Autodesk Inventor part; units mm, degrees
ref_plane "YZ Plane" through (0, 0, 0) normal (1, 0, 0) x (0, 1, 0)
ref_plane "XZ Plane" through (0, 0, 0) normal (0, 1, 0) x (-1, 0, 0)
ref_plane "XY Plane" through (0, 0, 0) normal (0, 0, 1) x (1, 0, 0)
sketch "Sketch1" plane through (0, 0, 0) normal (1, 0, 0) x (0, 1, 0)
  line L0 (0, 0) -> (800, 0)
  line L1 (800, 0) -> (800, -750)
  line L2 (800, -750) -> (0, -750)
  line L3 (0, -750) -> (0, 0)
  dimension "d0" = 800
  dimension "d1" = 750
extrude "Extrusion1" add sketch "Sketch1" along normal blind 18
sketch "Sketch2" plane through (18, 0, 0) normal (1, 0, 0) x (0, 0, -1)
  line L0 (0, 800) -> (0, 0)
  line L1 (750, 800) -> (0, 800)
  line L2 (400, 800) -> (418.5, 800)
  line L3 (418.5, 800) -> (418.5, 650)
  line L4 (418.5, 650) -> (400, 650)
  line L5 (400, 650) -> (400, 800)
  line L6 (0, 650) -> (300, 650)
  line L7 (300, 650) -> (300, 631.5)
  line L8 (300, 631.5) -> (0, 631.5)
  line L9 (0, 631.5) -> (0, 650)
  dimension "d4" = 400
  dimension "d5" = 18.5
  dimension "d6" = 150
  dimension "d7" = 300
  dimension "d8" = 18.5
extrude "Extrusion2" cut sketch "Sketch2" against normal blind 18
sketch "Sketch3" plane through (18, 0, 0) normal (1, 0, 0) x (0, 0, -1)
  circle A0 centre (50, 750) radius 5
  circle A1 centre (700, 750) radius 5
  circle A2 centre (700, 50) radius 5
  circle A3 centre (50, 50) radius 5
  point P0 (0, 0)
  point P1 (0, 800)
sketch "Sketch4" plane through (0, 800, -750) normal (0, 1, 0) x (1, 0, 0)
  circle A0 centre (0, -188) radius 5
  circle A1 centre (0, -375) radius 5
  circle A2 centre (0, -562) radius 5
  point P0 (0, -750)
  dimension "d25" = 10
  dimension "d26" = 10
  dimension "d27" = 10
extrude "Extrusion3" cut sketch "Sketch4" against normal blind 32
thread "Thread1"
thread "Thread2"
thread "Thread3"
sketch "Sketch5" plane through (0, 0, -750) normal (0, 0, -1) x (-1, 0, 0)
  line L0 (0, 0) -> (-9, 0)
  line L1 (0, 0) -> (-18, 0)
  circle A0 centre (-9, 600) radius 2.5
  circle A1 centre (-9, 200) radius 2.5
  circle A2 centre (-9, 400) radius 2.5
  dimension "d41" = 9
  dimension "d48" = 5
  dimension "d49" = 5
  dimension "d50" = 5
extrude "Extrusion4" cut sketch "Sketch5" against normal blind 18
extrude "Extrusion5" cut sketch "Sketch3" against normal blind 18
sketch "Sketch6" plane through (0, 0, 0) normal (-1, 0, 0) x (0, 0, 1)
  circle A0 centre (-300, 640.75) radius 2.5
  point P0 (0, 0)
  point P1 (-300, 631.5)
  dimension "d56" = 5
extrude "Extrusion6" cut sketch "Sketch6" against normal blind 18
sketch "Sketch7" plane through (18, 0, 0) normal (1, 0, 0) x (0, 0, -1)
  point P0 (0, 0)
sketch "Sketch8" plane through (18, 0, 0) normal (1, 0, 0) x (0, 0, -1)
  arc A0 (300, 638.25) -> (300, 643.25) centre (300, 640.75) ccw
  line L0 (300, 640.75) -> (409, 640.75) construction
  circle A1 centre (409, 640.75) radius 2.5
  circle A2 centre (409, 590.75) radius 2.5
  point P0 (0, 0)
  dimension "d62" = 5
  dimension "d63" = 5
extrude "Extrusion7" cut sketch "Sketch8" against normal blind 59.2125
sketch "Sketch9" plane through (18, 0, 0) normal (1, 0, 0) x (0, 0, -1)
  point P0 (0, 0)
properties part number "wallL1" material "MDF Medium Density Fiberboard"
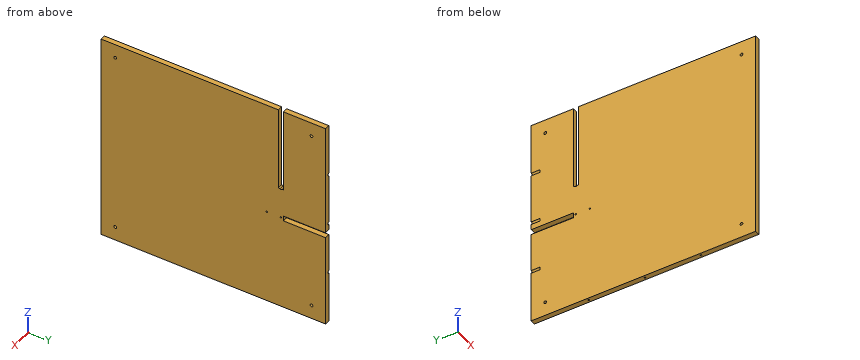
Check sheet for the modelled part. Datum: model origin and axes. Units: mm. Round coordinates to 2 decimals unless told otherwise and drop trailing zeros. Loops run counter-clockwise (first coordinate to the right, second up) from the corner with the lowest first, then second, coordinate; pieces in that order, holes last. Notation, with made-up numbers: M 72,24 L 76,24 A26 ccw 76,47 Z; hole C 63,73.25 d4. An arc over 180 degrees is marked long. One line per item, written item: value.
(1) Sectioned sample at A-A, the plane z = -142. Record the cut outline in (x, y).
Computed values:
outline: M 0,0 L 18,0 L 18,631.5 L 0,631.5 Z; M 0,650 L 18,650 L 18,800 L 0,800 Z
(2) Thickness scan on line 1 (Y direction, x = 8.5, z = -50); line 2 (Y direction, x = 9, z = -738); line 3 (Y direction, x = 8.75, z = -67). Record the ranges inside material, lowest first.
Computed values:
line 1: y = 0 to 45, 55 to 631.5, 650 to 745, 755 to 800
line 2: y = 0 to 197.5, 202.5 to 397.5, 402.5 to 597.5, 602.5 to 800
line 3: y = 0 to 631.5, 650 to 800
(3) Depth check by flat-ended pin: pin 1 Ø2 at (x, y) = (11.5, 647) entering from +Z; pin 2 Ø1.5 at (x, z) = (3.5, -190) entering from +Y; pin 3 Ø2.5 at (x, y) = (9.5, 400.5) entering from -Z. Enter the tip coordinate at first touch or a pass-through.
Computed values:
pin 1: stops at z = -300
pin 2: stops at y = 768
pin 3: stops at z = -732
